```python
from build123d import *

# Parameters (mm, degrees)
SKETCH2_R          = 2
CUT_EXTRUDE1_DEPTH = 10


with BuildPart() as part:
    # Sketch1 → Revolve1 (revolve)
    with BuildSketch(Plane(origin=(0, 0, 0), x_dir=(1, 0, 0), z_dir=(0, 1, 0)), mode=Mode.PRIVATE) as revolve1_sk:
        Polygon((-36.90300646, -9.632836954), (-13.12300646, -9.632836954), (-13.12300646, 25.367163046), (-26.90300646, 25.367163046), (-26.90300646, 29.367163046), (-33.90300646, 29.367163046), (-33.90300646, 42.367163046), (-36.90300646, 42.367163046), align=None)
    revolve(revolve1_sk.sketch.rotate(Axis((-36.90300646, 0, -63.116337875), (0, 0, 1)), 180), axis=Axis((-36.90300646, 0, -63.116337875), (0, 0, 1)))

    # Sketch2 → Cut-Extrude1 (cut)
    with BuildSketch(Plane(origin=(0, 0, -25.367163046), x_dir=(-1, 0, 0), z_dir=(0, 0, -1))):
        with Locations((25.40300646, 11.5)):
            Circle(SKETCH2_R)
        with Locations((48.40300646, 11.5)):
            Circle(SKETCH2_R)
        with Locations((48.40300646, -11.5)):
            Circle(SKETCH2_R)
        with Locations((25.40300646, -11.5)):
            Circle(SKETCH2_R)
    extrude(amount=-CUT_EXTRUDE1_DEPTH, mode=Mode.SUBTRACT)


solid = part.part
```
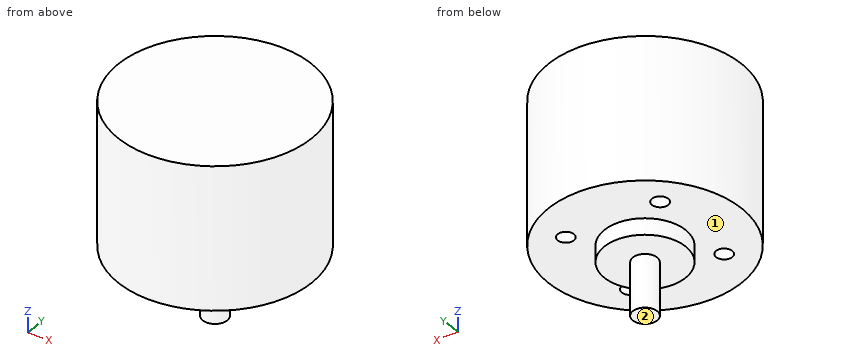
Input: part model. Units: mm. Frame: model coordinates. Face numbers are marked on the shaded views. A direction names the side the tool comes from. Coordinates: 2 decimals unless noted, no trailing zeros. Loops run counter-clockwise (first coordinate to the right, second up) from the corner with the lowest first, then second, coordinate; pieces in that order, holes last. Notation, with made-up numbers: M 46.25,-40 L 105.25,-40 A28 ccw 105.25,-11 Z; hole C 10.5,5.5 d6. An arc over 180 degrees is marked long. Use a Markdown table: item, result. Add a question column.
1) Section C-C, the plane z = -20.5. Return the cut outline in (x, y), plus the area to 3 significant figures.
2) Pin query (flat end, axial travel): P1, Ø5, axis at y = 16, z = -14, coming from the -X side; P2, Ø1.2, axis at x = -26.5, y = -11.5, coming from the -Z side; P3, Ø3, axis at y = 16, z = -26.5, coming from the -X side; P4, Ø16, axis at x = -36, y = -4.5, coming from the -Z side. Return the tip coordinate at first contact, or that it passes through.
3) Line query: L1, parallel to X at y = -11, z = -23; L2, parallel to Z at x = -56.5, y = -10.5; L3, parallel to Z at x = -31, y = -7. Output: solid intervals per line, ascending. Write a range as from..to.
4) Section D-D, the plane z = 4.5. Return the cut outline in (x, y), plus the area to 3 significant figures.
5) Section B-B, the plane x = -32. Return the cut outline in (y, z), plus the area to 3 significant figures.
6) Section A-A, the plane y = 0. Return the cut outline in (x, z), plus the area to 3 significant figures.
7) Set-up query: the marked faces 1 and 2. Return all of +Z, -Z, +X, -X, +Y, -Y with unobstructed straight access to the full face (end or side cutting, diameter ignored); none if empty.
Answer below:
| question | item | result |
|---|---|---|
| 1 | outline | C -36.9,0 d47.56; hole C -48.4,-11.5 d4; hole C -48.4,11.5 d4; hole C -25.4,-11.5 d4; hole C -25.4,11.5 d4 |
| 1 | area | 1,730 mm2 |
| 2 | P1 | x = -56.48 |
| 2 | P2 | z = -15.37 |
| 2 | P3 | x = -55.34 |
| 2 | P4 | z = -42.37 |
| 3 | L1 | -57.99..-50.34, -46.47..-27.34, -23.47..-15.82 |
| 3 | L2 | -25.37..9.63 |
| 3 | L3 | -29.37..9.63 |
| 4 | outline | C -36.9,0 d47.56 |
| 4 | area | 1,780 mm2 |
| 5 | outline | M -23.27,-25.37 L -8.72,-25.37 L -8.72,-29.37 L 8.72,-29.37 L 8.72,-25.37 L 23.27,-25.37 L 23.27,9.63 L -23.27,9.63 Z |
| 5 | area | 1,700 mm2 |
| 6 | outline | M -60.68,-25.37 L -46.9,-25.37 L -46.9,-29.37 L -39.9,-29.37 L -39.9,-42.37 L -33.9,-42.37 L -33.9,-29.37 L -26.9,-29.37 L -26.9,-25.37 L -13.12,-25.37 L -13.12,9.63 L -60.68,9.63 Z |
| 6 | area | 1,820 mm2 |
| 7 | face 1 | -Z |
| 7 | face 2 | -Z, +X, -X, +Y, -Y |
